from build123d import *

# Parameters (mm, degrees)
F0_R     = 1.7272
F0_R_2   = 3.96875
F0_R_3   = 9.525
F1_DEPTH = 3.175
F2_R     = 4.7625


with BuildPart() as f1:
    # F0 (on Top) → F1 (new body)
    with BuildSketch(Plane.XY):
        with BuildLine():
            Line((-303.612563, 32.54375), (-346.10942, 21.512003))
            ThreePointArc((-346.10942, 21.512003), (-362.750125, 0), (-346.10942, -21.512003))
            Line((-346.10942, -21.512003), (-303.612563, -32.54375))
            Line((-303.612563, -32.54375), (-297.262563, -32.54375))
            Line((-297.262563, -32.54375), (-297.262563, -29.36875))
            Line((-297.262563, -29.36875), (-43.262563, -29.36875))
            Line((-43.262563, -29.36875), (-43.262563, -32.54375))
            Line((-43.262563, -32.54375), (-36.912563, -32.54375))
            Line((-36.912563, -32.54375), (-16.771103, -27.315234))
            Line((-16.771103, -27.315234), (6.2453, -50.331637))
            ThreePointArc((6.2453, -50.331637), (7.790366, -51.364017), (9.612896, -51.726541))
            Line((9.612896, -51.726541), (70.052399, -51.726541))
            Line((70.052399, -51.726541), (70.052399, 51.726541))
            Line((70.052399, 51.726541), (9.612896, 51.726541))
            ThreePointArc((9.612896, 51.726541), (7.790366, 51.364017), (6.2453, 50.331637))
            Line((6.2453, 50.331637), (-16.771103, 27.315234))
            Line((-16.771103, 27.315234), (-36.912563, 32.54375))
            Line((-36.912563, 32.54375), (-43.262563, 32.54375))
            Line((-43.262563, 32.54375), (-43.262563, 29.36875))
            Line((-43.262563, 29.36875), (-297.262563, 29.36875))
            Line((-297.262563, 29.36875), (-297.262563, 32.54375))
            Line((-297.262563, 32.54375), (-303.612563, 32.54375))
        make_face()
        with Locations((-282.975063, -24.60625)):
            Circle(F0_R, mode=Mode.SUBTRACT)
        with Locations((-352.311712, -11.786586)):
            Circle(F0_R, mode=Mode.SUBTRACT)
        with Locations((-328.738539, -11.786586)):
            Circle(F0_R_2, mode=Mode.SUBTRACT)
        with Locations((9.612896, -46.964041)):
            Circle(F0_R, mode=Mode.SUBTRACT)
        with Locations((65.289899, -46.964041)):
            Circle(F0_R, mode=Mode.SUBTRACT)
        with Locations((-57.550063, -24.60625)):
            Circle(F0_R, mode=Mode.SUBTRACT)
        with Locations((0, -13.49375)):
            Circle(F0_R, mode=Mode.SUBTRACT)
        with Locations((-11.786586, -11.786586)):
            Circle(F0_R_2, mode=Mode.SUBTRACT)
        with Locations((11.786586, -11.786586)):
            Circle(F0_R, mode=Mode.SUBTRACT)
        with Locations((-340.525125, 0)):
            Circle(F0_R_3, mode=Mode.SUBTRACT)
        with Locations((-352.311712, 11.786586)):
            Circle(F0_R_2, mode=Mode.SUBTRACT)
        with Locations((-328.738539, 11.786586)):
            Circle(F0_R, mode=Mode.SUBTRACT)
        with Locations((-289.725125, 0)):
            Circle(F0_R, mode=Mode.SUBTRACT)
        with Locations((-282.975063, 24.60625)):
            Circle(F0_R, mode=Mode.SUBTRACT)
        with Locations((-50.8, 0)):
            Circle(F0_R, mode=Mode.SUBTRACT)
        with Locations((-57.550063, 24.60625)):
            Circle(F0_R, mode=Mode.SUBTRACT)
        Circle(F0_R_2, mode=Mode.SUBTRACT)
        with Locations((-11.786586, 11.786586)):
            Circle(F0_R, mode=Mode.SUBTRACT)
        with Locations((11.786586, 11.786586)):
            Circle(F0_R_2, mode=Mode.SUBTRACT)
        with Locations((0, 13.49375)):
            Circle(F0_R, mode=Mode.SUBTRACT)
        with Locations((9.612896, 46.964041)):
            Circle(F0_R, mode=Mode.SUBTRACT)
        with Locations((65.289899, 46.964041)):
            Circle(F0_R, mode=Mode.SUBTRACT)
    extrude(amount=F1_DEPTH)

    # F2
    f2_edges = [f1.edges().sort_by_distance(p)[0] for p in [
        (70.052399, 51.726541, 1.5875),
        (70.052399, -51.726541, 1.5875),
    ]]
    fillet(f2_edges, radius=F2_R)


solid = f1.part
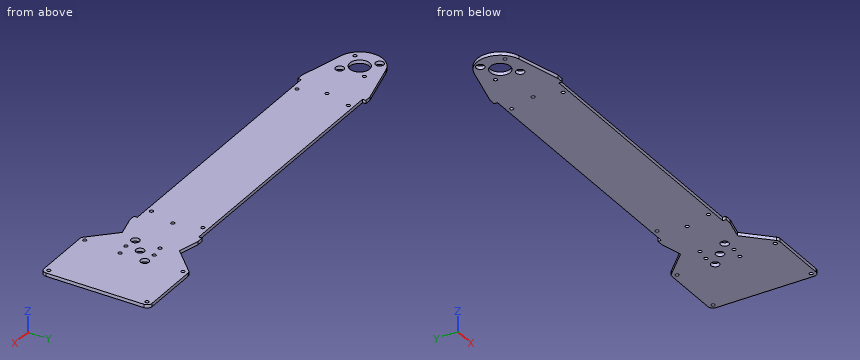
For this review, take the finished solid that the model builds, in its own axes (mm). Round coordinates to 2 decimals unless told otherwise and drop trailing zeros. Loops run counter-clockwise (first coordinate to the right, second up) from the corner with the lowest first, then second, coordinate; pieces in that order, holes last. Notation, with made-up numbers: (67.25, -17) - (76.25, -17) arc R20 ccw to (76.25, 16) - close; hole circle Ø10 at (27.25, -12). An arc over 180 degrees is marked (long way). Use one line per item in the form item = value.
Item 1: Consider section B-B on y = -40. Write out the cut boundary in (x, z) (3 decimals).
Answers:
outline = (-4.086, 0) - (70.052, 0) - (70.052, 3.175) - (-4.086, 3.175) - close
Item 2: Consider section C-C on z = 1.25. State how many separate pieces and enclosed holes the cut face has, then the cut area to 3 significant figures.
Answers:
separate_pieces = 1
enclosed_holes = 22
area = 27,500 mm^2
Item 3: Consider section A-A on x = -160.5. Write out the cut boundary in (y, z) (3 decimals), then the cut area to 3 significant figures.
Answers:
outline = (-29.369, 0) - (29.369, 0) - (29.369, 3.175) - (-29.369, 3.175) - close
area = 186 mm^2
Item 4: Clearance check with flat-ended pins moving along their axes: P1, Ø2, axis at x = -50.8, y = 0, coming from the -Z side; P2, Ø4, axis at x = 65.29, y = 46.96, coming from the -Z side; P3, Ø1, axis at x = -38.5, z = 1, coming from the -Y side; P4, Ø1, axis at x = -180, z = 0.5, coming from the +Y side. State where each tip first meets the part, or that it passes through.
Answers:
P1 = through
P2 = 0
P3 = -32.54
P4 = 29.37
Item 5: For line 1 (Y direction, x = -284.5, z = 1); line 2 (X direction, y = 47.5, z = 1.95); line 3 (Y direction, x = -1.5, z = 1.2), list the stretches that pass through material, from the lowest coordinate up.
Answers:
line_1 = -29.37 to -25.42, -23.8 to 23.8, 25.42 to 29.37
line_2 = 3.41 to 7.97, 11.25 to 63.65, 66.93 to 70.02
line_3 = -42.59 to -14.35, -12.64 to -3.67, 3.67 to 12.64, 14.35 to 42.59
